```python
from build123d import *

# Parameters (mm, degrees)
SKETCH1_R           = 22.5
BOSS_EXTRUDE1_DEPTH = 60
BOSS_EXTRUDE2_DEPTH = 98.836337037
SKETCH6_R           = 7.5
CUT_EXTRUDE1_DEPTH  = 159.836337037
CUT_EXTRUDE2_DEPTH  = 50


with BuildPart() as part:
    # Sketch1 → Boss-Extrude1 (new body)
    with BuildSketch(Plane.XY):
        Circle(SKETCH1_R)
    extrude(amount=BOSS_EXTRUDE1_DEPTH)

    # Sketch4 → Boss-Extrude2 (add)
    with BuildSketch(Plane(origin=(0, 0, 0), x_dir=(-1, 0, 0), z_dir=(0, 0, -1))):
        with BuildLine():
            Line((-2.5, 12.5), (2.5, 12.5))
            ThreePointArc((2.5, 12.5), (9.571067812, 9.571067812), (12.5, 2.5))
            Line((12.5, 2.5), (12.5, -2.5))
            ThreePointArc((12.5, -2.5), (9.571067812, -9.571067812), (2.5, -12.5))
            Line((2.5, -12.5), (-2.5, -12.5))
            ThreePointArc((-2.5, -12.5), (-9.571067812, -9.571067812), (-12.5, -2.5))
            Line((-12.5, -2.5), (-12.5, 2.5))
            ThreePointArc((-12.5, 2.5), (-9.571067812, 9.571067812), (-2.5, 12.5))
        make_face()
    extrude(amount=BOSS_EXTRUDE2_DEPTH)

    # Sketch5 → Revolve1 (revolve)
    with BuildSketch(Plane(origin=(0, 0, 0), x_dir=(0, 0, -1), z_dir=(1, 0, 0))):
        Polygon((-60, 106.5), (-60, 106.203428035), (-50.035306186, 22.5), (-45, 22.5), (-55, 106.5), align=None)
    revolve(axis=Axis((0, 0, 60), (0, 0, -1)))

    # Sketch6 → Cut-Extrude1 (cut, through all)
    with BuildSketch(Plane(origin=(0, 0, -98.836337037), x_dir=(-1, 0, 0), z_dir=(0, 0, -1))):
        Circle(SKETCH6_R)
    extrude(amount=-CUT_EXTRUDE1_DEPTH, mode=Mode.SUBTRACT)

    # Sketch7 → Cut-Extrude2 (cut)
    with BuildSketch(Plane.XY.offset(60)):
        with BuildLine():
            ThreePointArc((1.5, -7.348469228), (0, -7.5), (-1.5, -7.348469228))
            Line((-1.5, -7.348469228), (-1.5, -9.886859967))
            Line((-1.5, -9.886859967), (1.5, -9.886859967))
            Line((1.5, -9.886859967), (1.5, -7.348469228))
        make_face()
    extrude(amount=-CUT_EXTRUDE2_DEPTH, mode=Mode.SUBTRACT)


solid = part.part
```
Read the model definition and answer for the solid it produces. Units are mm, in the model's axes. A direction names the side the tool comes from. Coordinates: 2 decimals unless noted, no trailing zeros. Loops run counter-clockwise (first coordinate to the right, second up) from the corner with the lowest first, then second, coordinate; pieces in that order, holes last. Notation, with made-up numbers: (73.25, -19) - (114.25, -19) arc R20 ccw to (114.25, 3) - close; hole circle Ø7 at (61.25, -4.75). An arc over 180 degrees is marked (long way). Answer in a Markdown table with one row per item.
1. Determine the mould class of faces 1 (the face through (9.65, 9.49, -48.73)), 2 (the face through (21.46, 6.76, 54.95)), 3 (the face through (21.46, 6.76, 22.18)), 4 (the face through (7.493, 0.33, -20.53)) for opening direction Y: +Y half, -Y half, draft (parallel to the pull), parting line (faces both ways), or undercut.
Conclusion:
| item | result |
|---|---|
| face 1 | +Y half |
| face 2 | undercut |
| face 3 | parting line |
| face 4 | undercut |
2. Find section A-A, the plane z = -76. Write down the section's boundary in (x, y).
Conclusion:
| item | result |
|---|---|
| outline | (-12.5, -2.5) arc R10 ccw to (-2.5, -12.5) - (2.5, -12.5) arc R10 ccw to (12.5, -2.5) - (12.5, 2.5) arc R10 ccw to (2.5, 12.5) - (-2.5, 12.5) arc R10 ccw to (-12.5, 2.5) - close; hole circle Ø15 at (0, 0) |
3. Straight lines are drawn through the part: line 1 (X direction, y = 0, z = -47); line 2 (X direction, y = 0, z = 4). For each, find the intervals that lie inside material, in ascending order.
Conclusion:
| item | result |
|---|---|
| line 1 | x = -12.5 to -7.5, 7.5 to 12.5 |
| line 2 | x = -22.5 to -7.5, 7.5 to 22.5 |
4. Given pin 1 (2.5 mm diameter, centred on y = -1, z = -44, fed in from +X); pin 2 (1.3 mm diameter, centred on y = -8, z = 36.5, fed in from -X); pin 3 (5.5 mm diameter, centred on x = -1, z = -68, fed in from -Y), each flat-ended and moving along its own axis, determine where each tip first touches the part or whether it passes through.
Conclusion:
| item | result |
|---|---|
| pin 1 | stops at x = 12.5 |
| pin 2 | stops at x = -21.27 |
| pin 3 | stops at y = -12.5 |
5. Find section B-B, the plane z = 3.5. Write down the section's boundary in (x, y).
Conclusion:
| item | result |
|---|---|
| outline | circle Ø45 at (0, 0); hole circle Ø15 at (0, 0) |
6. Which of the six approach directions +Z, -Z, +X, -X, +Y, -Y give full straight-line access (tool end or side, diameter ignored) to faces 5 (the face through (10, 0, 60)), 6 (the face through (-9.49, 9.65, -48.73)), 7 (the face through (-9.65, -9.49, -48.73)), 8 (the face through (9.49, -9.65, -48.73)), 9 (the face through (10, -10, 0))?
Conclusion:
| item | result |
|---|---|
| face 5 | +Z, +X, -X, +Y, -Y |
| face 6 | -Z, -X, +Y |
| face 7 | -Z, -X, -Y |
| face 8 | -Z, +X, -Y |
| face 9 | -Z |
